Could you check a few things on this model? Use its own coordinates, in mm. Give positions to 0.01 mm unless a question says otherwise; leave off trailing zeros. Order: outer loops, then holes, each group sorted by start corner. A loop starts at its lowest first (then second) coordinate and runs counter-clockwise, first axis right, second up. Notation, with made-up numbers: M 37.25,-32.75 L 64.25,-32.75 A33 ccw 64.25,1.25 Z; hole C -11.75,8 d9. An arc over 180 degrees is marked long. Use a Markdown table: item, result. Add a question column.
Item 1: Suppose I cut it at B-B on y = 35. Write out the boundary of the cut face in (x, z).
Item 2: I'm going to push a flat-ended pin straight in: pin 1 Ø4 at (x, y) = (-59.944, 7.874) entering from +Z (3 decimals). Where does the tip first touch, or does it pass through?
Item 3: If I drill on L1, parallel to X at y = 35, z = 4; L2, parallel to Y at x = -8, z = 0.75; L3, parallel to Y at x = -72.5, z = 0.5, over which ranges is the centre line in solid material (lowest first)? Write a range as from..to.
Item 4: Suppose I cut it at C-C on z = 1.25. Count the separate pieces of the cut face and the enclosed holes in it, plus the area to 3 significant figures.
Item 5: Suppose I cut it at A-A on x = -31.56. Write out the boundary of the cut face in (y, z).
from build123d import *

# Parameters (mm, degrees)
SKETCH5_W               = 88.55
SKETCH5_H               = 69.55
SKETCH5_R               = 2.3876
SKETCH5_R_2             = 3.683
SKETCH5_R_3             = 4.953
SKETCH5_W_2             = 8.85
SKETCH5_H_2             = 31.2
SKETCH5_R_4             = 1.5875
BOSS_EXTRUDE1_DEPTH     = 6.35
F_8_32_TAPPED_HOLE1_D   = 3.4544
CUT_EXTRUDE2_START      = 3.175
SKETCH5_3_R             = 2.3876
SKETCH5_3_R_2           = 1.5875
CUT_EXTRUDE2_DEPTH      = 3.175
SKETCH8_W               = 25.4
SKETCH8_H               = 69.55
SKETCH8_R               = 1
BOSS_EXTRUDE2_DEPTH     = 6.35
F_1_4_20_TAPPED_HOLE2_D = 5.1054


with BuildPart() as part:
    # Sketch5 → Boss-Extrude1 (new body)
    # profile 1 of 6: a face of its own
    with BuildSketch(Plane.XY):
        with Locations((-47.069, 37.569)):
            Rectangle(SKETCH5_W, SKETCH5_H)
        with Locations((-7.874, 18.034)):
            Circle(SKETCH5_R, mode=Mode.SUBTRACT)
        with Locations((-7.874, 59.944)):
            Circle(SKETCH5_R, mode=Mode.SUBTRACT)
        with Locations((-18.034, 7.874)):
            Circle(SKETCH5_R, mode=Mode.SUBTRACT)
        with Locations((-59.944, 7.874)):
            Circle(SKETCH5_R, mode=Mode.SUBTRACT)
        with Locations((-19.9136, 19.9136)):
            Circle(SKETCH5_R_2, mode=Mode.SUBTRACT)
        with Locations((-49.594, 44.594)):
            Circle(SKETCH5_R_3, mode=Mode.SUBTRACT)
        with Locations((-74.919, 44.594)):
            Rectangle(SKETCH5_W_2, SKETCH5_H_2, mode=Mode.SUBTRACT)
        with Locations((-24.269, 44.594)):
            Rectangle(SKETCH5_W_2, SKETCH5_H_2, mode=Mode.SUBTRACT)
    # profile 2 of 6: a face of its own
    with BuildSketch(Plane.XY):
        with Locations((-7.874, 59.944)):
            Circle(SKETCH5_R)
        with Locations((-7.874, 59.944)):
            Circle(SKETCH5_R_4, mode=Mode.SUBTRACT)
    # profile 3 of 6: a face of its own
    with BuildSketch(Plane.XY):
        with Locations((-19.9136, 19.9136)):
            Circle(SKETCH5_R_2)
    # profile 4 of 6: a face of its own
    with BuildSketch(Plane.XY):
        with Locations((-7.874, 18.034)):
            Circle(SKETCH5_R)
        with Locations((-7.874, 18.034)):
            Circle(SKETCH5_R_4, mode=Mode.SUBTRACT)
    # profile 5 of 6: a face of its own
    with BuildSketch(Plane.XY):
        with Locations((-18.034, 7.874)):
            Circle(SKETCH5_R)
        with Locations((-18.034, 7.874)):
            Circle(SKETCH5_R_4, mode=Mode.SUBTRACT)
    # profile 6 of 6: a face of its own
    with BuildSketch(Plane.XY):
        with Locations((-59.944, 7.874)):
            Circle(SKETCH5_R)
        with Locations((-59.944, 7.874)):
            Circle(SKETCH5_R_4, mode=Mode.SUBTRACT)
    extrude(amount=BOSS_EXTRUDE1_DEPTH)

    # #8-32 Tapped Hole1 (through all)
    with Locations(Plane(origin=(-67.628, 44.594, 6.35), x_dir=(1, 0, 0), z_dir=(0, 0, 1))):
        with Locations((0, 0), (36.068, 0)):
            Hole(F_8_32_TAPPED_HOLE1_D / 2)

    # Sketch5<3> → Cut-Extrude2 (cut)
    # profile 1 of 4: a face of its own
    with BuildSketch(Plane.XY.offset(CUT_EXTRUDE2_START)):
        with Locations((-18.034, 7.874)):
            Circle(SKETCH5_3_R)
        with Locations((-18.034, 7.874)):
            Circle(SKETCH5_3_R_2, mode=Mode.SUBTRACT)
    # profile 2 of 4: a face of its own
    with BuildSketch(Plane.XY.offset(CUT_EXTRUDE2_START)):
        with Locations((-7.874, 18.034)):
            Circle(SKETCH5_3_R)
        with Locations((-7.874, 18.034)):
            Circle(SKETCH5_3_R_2, mode=Mode.SUBTRACT)
    # profile 3 of 4: a face of its own
    with BuildSketch(Plane.XY.offset(CUT_EXTRUDE2_START)):
        with Locations((-59.944, 7.874)):
            Circle(SKETCH5_3_R)
        with Locations((-59.944, 7.874)):
            Circle(SKETCH5_3_R_2, mode=Mode.SUBTRACT)
    # profile 4 of 4: a face of its own
    with BuildSketch(Plane.XY.offset(CUT_EXTRUDE2_START)):
        with Locations((-7.874, 59.944)):
            Circle(SKETCH5_3_R)
        with Locations((-7.874, 59.944)):
            Circle(SKETCH5_3_R_2, mode=Mode.SUBTRACT)
    extrude(amount=CUT_EXTRUDE2_DEPTH, mode=Mode.SUBTRACT)

    # Sketch8 → Boss-Extrude2 (add)
    with BuildSketch(Plane.XY):
        with Locations((-104.044, 37.569)):
            Rectangle(SKETCH8_W, SKETCH8_H)
        with Locations((-109.744, 7.794)):
            Circle(SKETCH8_R, mode=Mode.SUBTRACT)
    extrude(amount=BOSS_EXTRUDE2_DEPTH)

    # 1/4-20 Tapped Hole2 (through all)
    with Locations(Plane(origin=(-109.744, 7.794, 6.35), x_dir=(1, 0, 0), z_dir=(0, 0, 1))):
        with Locations((0, 0)):
            Hole(F_1_4_20_TAPPED_HOLE2_D / 2)


solid = part.part
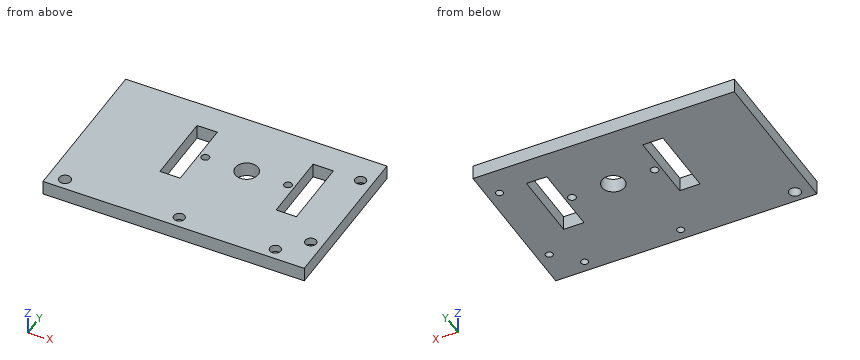
Findings below:
| question | item | result |
|---|---|---|
| 1 | outline | M -116.74,0 L -79.34,0 L -79.34,6.35 L -116.74,6.35 Z; M -70.49,0 L -28.69,0 L -28.69,6.35 L -70.49,6.35 Z; M -19.84,0 L -2.79,0 L -2.79,6.35 L -19.84,6.35 Z |
| 2 | pin 1 | stops at z = 3.175 |
| 3 | L1 | x = -116.74..-79.34, -70.49..-28.69, -19.84..-2.79 |
| 3 | L2 | y = 2.79..16.45, 19.62..58.36, 61.53..72.34 |
| 3 | L3 | y = 2.79..28.99, 60.19..72.34 |
| 4 | separate pieces | 1 |
| 4 | enclosed holes | 10 |
| 4 | area | 7,230 mm^2 |
| 5 | outline | M 2.79,0 L 42.87,0 L 42.87,6.35 L 2.79,6.35 Z; M 46.32,0 L 72.34,0 L 72.34,6.35 L 46.32,6.35 Z |
